Here's how the part is built. I have some questions about the finished solid (model axes, mm). A direction names the side the tool comes from. Coordinates: 2 decimals unless noted, no trailing zeros. Loops run counter-clockwise (first coordinate to the right, second up) from the corner with the lowest first, then second, coordinate; pieces in that order, holes last. Notation, with made-up numbers: (-9, 67) -> (15, 67) arc R30 ccw to (15, 99) -> close; hole circle Ø2 at (24.5, 81). An arc over 180 degrees is marked (long way). Answer as a JSON object with one key per item and string values. Group by question number.
Q1. I need wall thicknesses on line 1 (X direction, y = -14, z = -36); line 2 (Y direction, x = 41, z = -163.5); line 3 (Y direction, x = -8.5, z = -91). Which ranges of each line are inside material? Lowest first, please.
Q2. I want a section at A-A on x = -21.5. Write out the boundary of the cut face in (y, z), then the cut area to 3 significant figures.
Q3. I'm going to push flat-ended pins straight in: pin 1 (2 mm diameter, centred on y = -25.5, z = 82.5, fed in from -X); pin 2 (2 mm diameter, centred on x = -31, z = 55, fed in from +Y); pin 3 (12 mm diameter, centred on x = 12, y = -7.5, fed in from -Z); pin 4 (1 mm diameter, centred on y = -9.5, z = -154, fed in from +X). Where does each tip first touch, or does it pass through?
Q4. I want a section at B-B on z = -29.5. Write out the boundary of the cut face in (x, y).
Q5. Thinking about a two-plate mould opening in Z: for faces 5 (the flat face through (46.228, -5, -140)), 6 (the flat face through (0.647, -1.194, -187.218)), 7 (the cylindrical face through (-31.555, -26.796, 86.088)), which applies, released by +Z, released by -Z, zero draft, split by the parting line, or undercut?
Q6. On a 3-axis mill with a long thin cutter (end or side, diameter ignored), from which of +Z, -Z, +X, -X, +Y, -Y can I reach the whole of each face in a straight line? I mean faces 1 (the flat face through (-43.477, -28.817, 106.404)), 2 (the flat face through (25.4, -19, 5)), 3 (the flat face through (-0.356, -22.73, 44.493)), 4 (the flat face through (41.21, -1.93, -155.32)). Say none if no direction works.
Q7. I want a section at C-C on z = -75. Write out the boundary of the cut face in (x, y).
```python
from build123d import *

# Parameters (mm, degrees)
FRAME_DEPTH              = 46.228
SKETCH7_W                = 50.8
SKETCH7_H                = 81.247188803
BATTERY_SLOT_DEPTH       = 32.131
EXTRUDE25_DEPTH          = 12.7
LOW_A_ARM_MOUNTING_DEPTH = 8.128
REAR_HINGE_HOLES_REACH   = 309.358
SKETCH25_R               = 1.905
SKETCH33_R               = 3.175
EXTRUDE23_DEPTH          = 9.652
SKETCH32_R               = 3.175
EXTRUDE24_DEPTH          = 9.652
SKETCH34_R               = 1.905
EXTRUDE26_DEPTH          = 40.894


with BuildPart() as part:
    # Sketch2 → Frame (new, symmetric)
    with BuildSketch(Plane(origin=(0, 0, 0), x_dir=(0, 0, -1), z_dir=(1, 0, 0))):
        Polygon((-113.716301345, -32.469135694), (-63.34929575, -27.768288573), (187.512811896, -4.354857448), (186.914499493, 2.05573268), (-66.485612868, -21.594575186), (-114.265856874, -26.580948798), align=None)
    extrude(amount=FRAME_DEPTH, both=True)

    # Sketch7 → Battery Slot (cut)
    with BuildSketch(Plane(origin=(0, -15.256451714, -1.42391326), x_dir=(1, 0, 0), z_dir=(0, 0.9956728299897474, 0.09292801310803929))):
        with Locations((0, -5.788843516)):
            Rectangle(SKETCH7_W, SKETCH7_H)
    extrude(amount=-BATTERY_SLOT_DEPTH, mode=Mode.SUBTRACT)

    # Sketch20 → Extrude25 (cut)
    with BuildSketch(Plane(origin=(0, -21.667041842, -2.022225663), x_dir=(1, 0, 0), z_dir=(0, -0.9956728299897474, -0.09292801310803922))):
        Polygon((54.692263435, 108.621523843), (36.068, 108.621523843), (36.068, 98.461523843), (48.857667711, 98.461523843), (48.857667711, 88.301523843), (36.068, 88.301523843), (36.068, 78.141523843), (53.624725675, 78.141523843), align=None)
        Polygon((-53.624725675, 78.141523843), (-54.692263435, 108.621523843), (-36.068, 108.621523843), (-36.068, 98.461523843), (-48.857667711, 98.461523843), (-48.857667711, 88.301523843), (-36.068, 88.301523843), (-36.068, 78.141523843), align=None)
    extrude(amount=-EXTRUDE25_DEPTH, mode=Mode.SUBTRACT)

    # Sketch24 → Low A-Arm Mounting (cut)
    with BuildSketch(Plane(origin=(0, -15.256451714, -1.42391326), x_dir=(1, 0, 0), z_dir=(0, 0.9956728299897474, 0.09292801310803929))):
        Polygon((56.409110401, 123.988548499), (56.409110401, 154.468520321), (36.047664653, 154.468520321), (36.061546605, 144.259475636), (46.249110401, 144.259475636), (46.249110401, 134.050421513), (36.07522845, 134.197593184), (36.089110401, 123.988548499), align=None)
        Polygon((-36.089110402, 123.939475636), (-56.409091616, 123.911845137), (-56.450537326, 154.39178878), (-36.089110402, 154.419475636), (-36.089110402, 144.210421513), (-46.27666478, 144.196568783), (-46.262782828, 133.987524098), (-36.089110402, 134.148529759), align=None)
    extrude(amount=-LOW_A_ARM_MOUNTING_DEPTH, mode=Mode.SUBTRACT)

    # Rear Hinge Holes: up to this face of the body (flat: up to its plane)
    rear_hinge_holes_end = Plane(part.part.faces().sort_by_distance((41.158555201, -6.939737318, -125.175098432))[0])
    # Sketch25 → Rear Hinge Holes (cut, up to the picked face)
    with BuildSketch(Plane(origin=(0, 17.312184394, -185.490586234), x_dir=(-1, 0, 0), z_dir=(0, 0.09292801310803887, -0.9956728299897473)), mode=Mode.PRIVATE) as rear_hinge_holes_sk1:
        with Locations(Location((-41.073322363, -18.541981083, 0), (0, 0, 90))):
            Circle(SKETCH25_R)
    rear_hinge_holes_tool1 = split(extrude(rear_hinge_holes_sk1.sketch, amount=-REAR_HINGE_HOLES_REACH, mode=Mode.PRIVATE), bisect_by=rear_hinge_holes_end, keep=Keep.BOTH, mode=Mode.PRIVATE)
    # Sketch25 → Rear Hinge Holes (cut, up to the picked face)
    with BuildSketch(Plane(origin=(0, 17.312184394, -185.490586234), x_dir=(-1, 0, 0), z_dir=(0, 0.09292801310803887, -0.9956728299897473)), mode=Mode.PRIVATE) as rear_hinge_holes_sk2:
        with Locations(Location((41.073322363, -18.541981083, 0), (0, 0, 180))):
            Circle(SKETCH25_R)
    rear_hinge_holes_tool2 = split(extrude(rear_hinge_holes_sk2.sketch, amount=-REAR_HINGE_HOLES_REACH, mode=Mode.PRIVATE), bisect_by=rear_hinge_holes_end, keep=Keep.BOTH, mode=Mode.PRIVATE)
    add(rear_hinge_holes_tool1.solids().sort_by(Axis((41.073322, -1.149562, -187.213656), (0, -0.09292801310803887, 0.9956728299897473)))[0], mode=Mode.SUBTRACT)
    add(rear_hinge_holes_tool2.solids().sort_by(Axis((-41.073322, -1.149562, -187.213656), (0, -0.09292801310803887, 0.9956728299897473)))[0], mode=Mode.SUBTRACT)

    # Sketch33 → Extrude23 (cut)
    with BuildSketch(Plane(origin=(0, -21.667041842, -2.022225663), x_dir=(1, 0, 0), z_dir=(0, -0.9956728299897473, -0.09292801310803925))):
        with Locations(Location((28.407237147, -144.13272383, 0), (0, 0, 270))):
            Circle(SKETCH33_R)
        with Locations(Location((-28.407237147, -144.13272383, 0), (0, 0, 270))):
            Circle(SKETCH33_R)
    extrude(amount=-EXTRUDE23_DEPTH, mode=Mode.SUBTRACT)

    # Sketch32 → Extrude24 (cut)
    with BuildSketch(Plane(origin=(0, -21.667041842, -2.022225663), x_dir=(1, 0, 0), z_dir=(0, -0.9956728299897473, -0.0929280131080392))):
        with Locations(Location((28.407237147, 88.619023843, 0), (0, 0, 270))):
            Circle(SKETCH32_R)
        with Locations(Location((-28.407237147, 88.619023843, 0), (0, 0, 90))):
            Circle(SKETCH32_R)
    extrude(amount=-EXTRUDE24_DEPTH, mode=Mode.SUBTRACT)

    # Sketch34 → Extrude26 (cut)
    with BuildSketch(Plane(origin=(0, -10.802093851, 115.738527007), x_dir=(1, 0, 0), z_dir=(0, -0.09292801310803855, 0.9956728299897473))):
        with Locations(Location((-41.073774155, -18.804317875, 0), (0, 0, 270))):
            Circle(SKETCH34_R)
        with Locations(Location((41.073774155, -18.804317875, 0), (0, 0, 270))):
            Circle(SKETCH34_R)
    extrude(amount=-EXTRUDE26_DEPTH, mode=Mode.SUBTRACT)


solid = part.part
```
Result set:
{
 "1": {"line 1": "x = -46.23 to -25.4, 25.4 to 46.23", "line 2": "y = -6.6 to -5.27, -1.45 to -0.13", "line 3": "y = -13.36 to -6.9"},
 "2": {"outline": "(-32.47, 113.72) -> (-25.98, 44.19) -> (-19.57, 44.79) -> (-21.59, 66.49) -> (-26.58, 114.27) -> close; (-18.43, -36.71) -> (-4.35, -187.51) -> (2.06, -186.91) -> (-12.02, -36.11) -> close", "area": "1,410 mm²"},
 "3": {"pin 1": "stops at x = -36.07", "pin 2": "stops at y = -20.43", "pin 3": "stops at z = -187.51", "pin 4": "passes through"},
 "4": {"outline": "(-46.23, -19.1) -> (-25.4, -19.1) -> (-25.4, -12.64) -> (-46.23, -12.64) -> close; (25.4, -19.1) -> (46.23, -19.1) -> (46.23, -12.64) -> (25.4, -12.64) -> close"},
 "5": {"face 5": "zero draft", "face 6": "released by -Z", "face 7": "undercut"},
 "6": {"face 1": "-X, +Y", "face 2": "+Y, -Y", "face 3": "-Z, +Y", "face 4": "+X, -Y"},
 "7": {"outline": "(-46.23, -14.86) -> (46.23, -14.86) -> (46.23, -8.39) -> (-46.23, -8.39) -> close"}
}
